Geometry check sheet. Reference: the model listing, model coordinates, mm. Face numbers are marked on the shaded views. Round coordinates to 2 decimals unless told otherwise and drop trailing zeros. Order: outer loops, then holes, each group sorted by start corner. A loop starts at its lowest first (then second) coordinate and runs counter-clockwise, first axis right, second up.
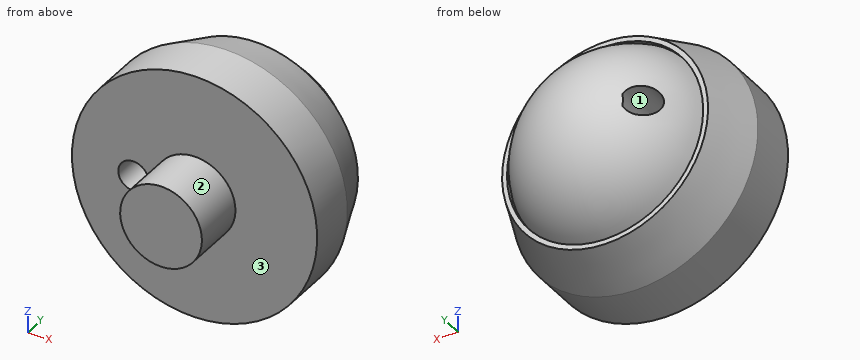
```python
from build123d import *

# Parameters (mm, degrees)
ECHELLE1_SCALE          = 0.6
ESQUISSE3_R             = 7.5
BOSS_EXTRU_1_DEPTH      = 10
ESQUISSE4_R             = 2.75
ENL_V_MAT_EXTRU_1_DEPTH = 27


with BuildPart() as part:
    # Esquisse2 → Révolution1 (revolve)
    with BuildSketch(Plane.XY, mode=Mode.PRIVATE) as r_volution1_sk:
        with BuildLine():
            Line((0, 0), (37.5, 0))
            Line((37.5, 0), (37.5, 15))
            Line((37.5, 15), (31.5, 30))
            Line((31.5, 30), (30, 30))
            Line((30, 30), (30, 28.5))
            ThreePointArc((30, 28.5), (18.027756377, 43.041634566), (0, 48.5))
            Line((0, 48.5), (0, 0))
        make_face()
    revolve(r_volution1_sk.sketch.rotate(Axis((0, 0, 0), (0, 1, 0)), 90), axis=Axis((0, 0, 0), (0, 1, 0)))


with BuildPart() as part_1:
    # Echelle1: scaled about (0, 0, 0)
    add(part.part.scale(ECHELLE1_SCALE))

    # Esquisse3 → Boss.-Extru.1 (add)
    with BuildSketch(Plane(origin=(0, 0, 0), x_dir=(-1, 0, 0), z_dir=(0, -1, 0))):
        with Locations(Location((0, 0, 0), (0, 0, 90))):
            Circle(ESQUISSE3_R)
    extrude(amount=BOSS_EXTRU_1_DEPTH)

    # Esquisse4 → Enlèv. mat.-Extru.1 (cut)
    with BuildSketch(Plane(origin=(0, 0, 0), x_dir=(-1, 0, 0), z_dir=(0, -1, 0))):
        with Locations(Location((11.25, 0, 0), (0, 0, 90))):
            Circle(ESQUISSE4_R)
    extrude(amount=-ENL_V_MAT_EXTRU_1_DEPTH, mode=Mode.SUBTRACT)


solid = part_1.part
```
(1) Draft check along Z on the marked faces 1, 2 and 3. Enter one of: released by +Z, released by -Z, zero draft, split by the parting line, or undercut.
Returned:
face 1: undercut
face 2: split by the parting line
face 3: zero draft
(2) Depth check by flat-ended pin: P1, Ø5, axis at y = 4.5, z = 13, coming from the -X side; P2, Ø1, axis at y = 3.5, z = -16, coming from the +X side; P3, Ø10, axis at x = -4, y = -4.5, coming from the +Z side. Enter the tip coordinate at first touch or a pass-through.
Returned:
P1: stops at x = -19.9
P2: stops at x = 16.31
P3: stops at z = 22.43
(3) Material ranges on line 1 (X direction, y = 17.5, z = -9); line 2 (X direction, y = 5.5, z = 0); line 3 (Z direction, x = -11, y = 6), recorded low to high.
Returned:
line 1: x = -16.85 to -15.59, -15.39 to 15.39, 15.59 to 16.85
line 2: x = -22.5 to -14, -8.5 to 22.5
line 3: z = -19.63 to -2.74, 2.74 to 19.63
(4) Sectioned sample at A-A, the plane x = 0. Record the cut outline in (y, z).
Returned:
outline: (-10, -7.5) - (0, -7.5) - (0, -22.5) - (9, -22.5) - (18, -18.9) - (18, -18) - (17.1, -18) arc R19.5 ccw to (17.1, 18) - (18, 18) - (18, 18.9) - (9, 22.5) - (0, 22.5) - (0, 7.5) - (-10, 7.5) - close
(5) Sectioned sample at B-B, the plane y = 2.5. Record the cut outline in (x, z), and give its area (3 significant figures).
Returned:
outline: circle Ø45 at (0, 0); hole circle Ø5.5 at (-11.25, 0)
area: 1,570 mm2
